```python
from build123d import *

# Parameters (mm, degrees)
SKETCH1_W           = 40
SKETCH1_H           = 20
BOSS_EXTRUDE1_DEPTH = 5
SKETCH2_R           = 8
BOSS_EXTRUDE2_DEPTH = 10
BOSS_EXTRUDE3_DEPTH = 20
CUT_EXTRUDE1_DEPTH  = 42.952353927
SKETCH6_R           = 5
CUT_EXTRUDE2_DEPTH  = 53.763623833


with BuildPart() as part:
    # Sketch1 → Boss-Extrude1 (new body)
    with BuildSketch(Plane(origin=(0, 0, 0), x_dir=(1, 0, 0), z_dir=(0, 1, 0))):
        with Locations((20, 10)):
            Rectangle(SKETCH1_W, SKETCH1_H)
    extrude(amount=BOSS_EXTRUDE1_DEPTH)

    # Sketch2 → Boss-Extrude2 (add)
    with BuildSketch(Plane(origin=(0, 5, 0), x_dir=(1, 0, 0), z_dir=(0, 1, 0))):
        with Locations(Location((9.5, 10, 0), (0, 0, 270))):
            Circle(SKETCH2_R)
    extrude(amount=BOSS_EXTRUDE2_DEPTH)

    # Sketch4 → Boss-Extrude3 (add, through all)
    with BuildSketch(Plane.XY):
        Polygon((-6, 15), (0, 15), (1.5, 15), (17.5, 15), (18, 15), (18, 28), (-6, 28), align=None)
    extrude(amount=-BOSS_EXTRUDE3_DEPTH)

    # Sketch5 → Cut-Extrude1 (cut, through all)
    with BuildSketch(Plane(origin=(18, 0, 0), x_dir=(0, 0, -1), z_dir=(1, 0, 0))):
        Polygon((10, 15), (16, 15), (16, 28), (4, 28), (4, 15), align=None)
    extrude(amount=-CUT_EXTRUDE1_DEPTH, mode=Mode.SUBTRACT)

    # Sketch6 → Cut-Extrude2 (cut, through all)
    with BuildSketch(Plane.XY):
        with Locations((6, 21.5)):
            Circle(SKETCH6_R)
    extrude(amount=-CUT_EXTRUDE2_DEPTH, mode=Mode.SUBTRACT)


solid = part.part
```
CAD build for the part. Positions are in the model's coordinates, mm. A direction names the side the tool comes from. Give positions to 0.01 mm unless a question says otherwise; leave off trailing zeros. Order: outer loops, then holes, each group sorted by start corner. A loop starts at its lowest first (then second) coordinate and runs counter-clockwise, first axis right, second up.
(1) Saw through at B-B, the plane x = 7. Give the cut face in (y, z), then the cut area to 3 significant figures.
(2) Saw through at C-C, the plane z = -6.5. Give the cut face in (x, y), then the cut area to 3 significant figures.
(3) Saw through at A-A, the plane y = 18.5. Give the cut face in (x, z).
(4) Mould opens along Z. For faces 5 (the flat face through (10, 15, -10)), 6 (the cylindrical face through (4.92, 16.62, -1.97)), 7 (the flat face through (9, 17, -16)), 8 (the flat face through (20, 2, 0)) say: released by +Z, released by -Z, zero draft, split by the parting line, or undercut.
(5) Tool access for faces 1 (the flat face through (6, 15, -18)), 2 (the flat face through (9, 26, -4)), 3 (the cylindrical face through (4.92, 16.62, -17.97)), 4 (the flat face through (18, 21, -18)): list every direction of +Z, -Z, +X, -X, +Y, -Y with a clear straight run to the whole face (end or side of a thin tool).
(6) Drill centre lines: L1, parallel to Y at x = 6, z = -17.8; L2, parallel to Z at x = 13, y = 26.25; L3, parallel to Y at x = 37.5, z = -12.5. Where is each one in solid material? Low to high.
(7) Saw through at D-D, the plane y = 21.5. Give the cut face in (x, z), then the cut area to 3 significant figures.
(8) Flat gauge pins, fed straight in: pin 1 (6 mm diameter, centred on x = 5, y = 20.5, fed in from -Z); pin 2 (1.2 mm diameter, centred on y = 24, z = -2, fed in from +X); pin 3 (3.5 mm diameter, centred on x = 6.5, z = -12.5, fed in from +Y); pin 4 (6 mm diameter, centred on x = 25, z = -18, fed in from +Y). Where does each tip first touch, or does it go through?
Results found:
1. outline: (0, -20) - (5, -20) - (5, -17.6) - (15, -17.6) - (15, -20) - (16.6, -20) - (16.6, -16) - (15, -16) - (15, -4) - (16.6, -4) - (16.6, 0) - (15, 0) - (15, -2.4) - (5, -2.4) - (5, 0) - (0, 0) - close; (26.4, -20) - (28, -20) - (28, -16) - (26.4, -16) - close; (26.4, -4) - (28, -4) - (28, 0) - (26.4, 0) - close
1. area: 278 mm2
2. outline: (0, 0) - (40, 0) - (40, 5) - (16.69, 5) - (16.69, 15) - (2.31, 15) - (2.31, 5) - (0, 5) - close
2. area: 344 mm2
3. outline: (-6, -20) - (2, -20) - (2, -16) - (-6, -16) - close; (-6, -4) - (2, -4) - (2, 0) - (-6, 0) - close; (10, -20) - (18, -20) - (18, -16) - (10, -16) - close; (10, -4) - (18, -4) - (18, 0) - (10, 0) - close
4. face 5: undercut
4. face 6: zero draft
4. face 7: undercut
4. face 8: released by +Z
5. face 1: -Z
5. face 2: +X, -X, +Y
5. face 3: +Z, -Z
5. face 4: +Z, -Z, +X, +Y
6. L1: y = 0 to 5, 15 to 16.5, 26.5 to 28
6. L2: z = -20 to -16, -4 to 0
6. L3: y = 0 to 5
7. outline: (-6, -20) - (1, -20) - (1, -16) - (-6, -16) - close; (-6, -4) - (1, -4) - (1, 0) - (-6, 0) - close; (11, -20) - (18, -20) - (18, -16) - (11, -16) - close; (11, -4) - (18, -4) - (18, 0) - (11, 0) - close
7. area: 112 mm2
8. pin 1: passes through
8. pin 2: stops at x = 18
8. pin 3: stops at y = 15
8. pin 4: stops at y = 5
